from build123d import *

# Parameters (mm, degrees)
SKETCH1_R           = 1.5
BOSS_EXTRUDE1_DEPTH = 4.4
SKETCH2_R           = 2.75
BOSS_EXTRUDE2_DEPTH = 9.2
SKETCH3_R           = 5.925
BOSS_EXTRUDE3_DEPTH = 2.73
FILLET1_R           = 0.5
SKETCH4_R           = 4.925
CUT_EXTRUDE1_DEPTH  = 0.1


with BuildPart() as part:
    # Sketch1 → Boss-Extrude1 (new body)
    with BuildSketch(Plane(origin=(0, 0, 0), x_dir=(1, 0, 0), z_dir=(0, 1, 0))):
        with Locations(Location((0, 0, 0), (0, 0, 270))):
            Circle(SKETCH1_R)
    extrude(amount=BOSS_EXTRUDE1_DEPTH)

    # Sketch2 → Boss-Extrude2 (add)
    with BuildSketch(Plane(origin=(0, 4.4, 0), x_dir=(1, 0, 0), z_dir=(0, 1, 0))):
        with Locations(Location((0, 0, 0), (0, 0, 270))):
            Circle(SKETCH2_R)
    extrude(amount=BOSS_EXTRUDE2_DEPTH)

    # Sketch3 → Boss-Extrude3 (add)
    with BuildSketch(Plane(origin=(0, 13.6, 0), x_dir=(1, 0, 0), z_dir=(0, 1, 0))):
        with Locations(Location((0, 0, 0), (0, 0, 90))):
            Circle(SKETCH3_R)
    extrude(amount=BOSS_EXTRUDE3_DEPTH)

    # Fillet1
    fillet1_edges = [part.edges().sort_by_distance(p)[0] for p in [
        (0, 13.6, -2.75),
    ]]
    fillet(fillet1_edges, radius=FILLET1_R)

    # Sketch4 → Cut-Extrude1 (cut)
    with BuildSketch(Plane(origin=(0, 16.33, 0), x_dir=(1, 0, 0), z_dir=(0, 1, 0))):
        with Locations(Location((0, 0, 0), (0, 0, 270))):
            Circle(SKETCH4_R)
    extrude(amount=-CUT_EXTRUDE1_DEPTH, mode=Mode.SUBTRACT)


solid = part.part
The model under review builds one solid part; all positions refer to its coordinate system, in mm. A direction names the side the tool comes from. Round coordinates to 2 decimals unless told otherwise and drop trailing zeros. Loops run counter-clockwise (first coordinate to the right, second up) from the corner with the lowest first, then second, coordinate; pieces in that order, holes last. Notation, with made-up numbers: M 59.5,-11 L 105.5,-11 A20 ccw 105.5,7 Z; hole C 43.25,11.25 d11. An arc over 180 degrees is marked long. Answer as a JSON object with one key per item and string values.
Item 1: Clearance check with flat-ended pins moving along their axes: P1, Ø3, axis at x = -3, y = 5.5, coming from the +Z side; P2, Ø1.5, axis at y = 2.5, z = 0, coming from the +X side; P3, Ø1.5, axis at x = 4.5, y = 14, coming from the +Z side. State where each tip first meets the part, or that it passes through.
Check sheet entries:
{"P1": "z = 2.3", "P2": "x = 1.5", "P3": "z = 4.59"}
Item 2: We need section C-C, the plane y = 5. State the section outline as (x, z) points.
Check sheet entries:
{"outline": "C 0,0 d5.5"}
Item 3: We need section A-A, the plane x = 0. State the section outline as (y, z) points (3 decimals), and give its area (3 significant figures).
Check sheet entries:
{"outline": "M 0,-1.5 L 4.4,-1.5 L 4.4,-2.75 L 13.1,-2.75 A0.5 cw 13.6,-3.25 L 13.6,-5.925 L 16.33,-5.925 L 16.33,-4.925 L 16.23,-4.925 L 16.23,4.925 L 16.33,4.925 L 16.33,5.925 L 13.6,5.925 L 13.6,3.25 A0.5 cw 13.1,2.75 L 4.4,2.75 L 4.4,1.5 L 0,1.5 Z", "area": "95.3 mm2"}
Item 4: For line 1 along Y through (x, z) = (0.25, -4.75); line 2 along Y through (x, z) = (4.25, -3.5); line 3 along X through (y, z) = (15.25, -3), list the stretches that pass through material, from the lowest coordinate up.
Check sheet entries:
{"line 1": "13.6 to 16.23", "line 2": "13.6 to 16.33", "line 3": "-5.11 to 5.11"}
Item 5: We need section B-B, the plane z = 0. State the section outline as (x, y) points (3 decimals), and give its area (3 significant figures).
Check sheet entries:
{"outline": "M -5.925,13.6 L -3.25,13.6 A0.5 cw -2.75,13.1 L -2.75,4.4 L -1.5,4.4 L -1.5,0 L 1.5,0 L 1.5,4.4 L 2.75,4.4 L 2.75,13.1 A0.5 cw 3.25,13.6 L 5.925,13.6 L 5.925,16.33 L 4.925,16.33 L 4.925,16.23 L -4.925,16.23 L -4.925,16.33 L -5.925,16.33 Z", "area": "95.3 mm2"}
Item 6: We need section D-D, the plane y = 2. State the section outline as (x, z) points, and give its area (3 significant figures).
Check sheet entries:
{"outline": "C 0,0 d3", "area": "7.07 mm2"}
Item 7: Tool access review of faces 4 (the face through (0, 0, 0)), 5 (the face through (3, 13.6, -3)): name each direction out of +Z, -Z, +X, -X, +Y, -Y from which nothing blocks a thin tool from reaching the whole face with its end or side.
Check sheet entries:
{"face 4": "+Z, -Z, +X, -X, -Y", "face 5": "-Y"}
Item 8: The part is to be moulded in two halves that separate along X. For faces 1 (the face through (0, 16.23, 0)), 2 (the face through (-2.685, 8.689, -0.596)), 3 (the face through (-5, 16.33, -1)), say which applies: +X half, -X half, draft (parallel to the pull), parting line (faces both ways), or undercut.
Check sheet entries:
{"face 1": "undercut", "face 2": "parting line", "face 3": "draft"}
